Verification items for the finished model (mm, model axes). Face numbers are marked on the shaded views. A direction names the side the tool comes from. Round coordinates to 2 decimals unless told otherwise and drop trailing zeros. Write each loop counter-clockwise with the first axis right and the second up, starting at its lowest first coordinate (ties: lowest second). Pieces come first, ordered by that corner, then holes. Notation, with made-up numbers: (-5.75, 23) - (48.25, 23) arc R17 cw to (48.25, 39) - close; hole circle Ø7 at (83, -23). An arc over 180 degrees is marked (long way). Answer as a JSON object with one key per item and string values.
```python
from build123d import *

# Parameters (mm, degrees)
BOSS_EXTRUDE1_START = 7.7
SKETCH2_R           = 1.295
BOSS_EXTRUDE1_DEPTH = 7.7


with BuildPart() as part:
    # Sketch1 → Revolve1 (revolve)
    with BuildSketch(Plane.XY, mode=Mode.PRIVATE) as revolve1_sk:
        Polygon((-2.7, 0), (-2.7, 5.54), (-1.295, 5.54), (-1.295, 8.3), (-3.32, 8.3), (-3.97, 7.184383121), (-3.97, 3.67), (-4.785, 3.67), (-4.785, 2.47), (-4.28, 2.47), (-4.325, 0), align=None)
    revolve(revolve1_sk.sketch.rotate(Axis((0, 0, 0), (0, 1, 0)), 270), axis=Axis((0, 0, 0), (0, 1, 0)))

    # Sketch2 → Boss-Extrude1 (add)
    with BuildSketch(Plane(origin=(0, 8.3, 0), x_dir=(1, 0, 0), z_dir=(0, 1, 0)).offset(BOSS_EXTRUDE1_START)):
        Polygon((1.799527716, 2.79), (-1.799527716, 2.79), (-2.79, 1.799527716), (-2.79, -1.799527716), (-1.799527716, -2.79), (1.799527716, -2.79), (2.79, -1.799527716), (2.79, 1.799527716), align=None)
        with Locations(Location((0, 0, 0), (0, 0, 90))):
            Circle(SKETCH2_R, mode=Mode.SUBTRACT)
    extrude(amount=-BOSS_EXTRUDE1_DEPTH)


solid = part.part
```
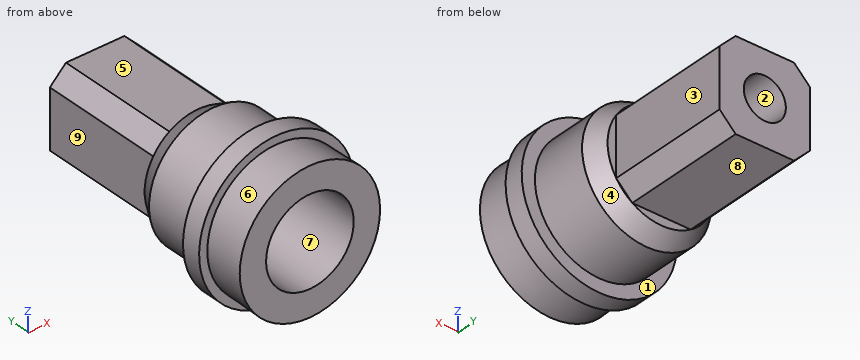
Q1. Section check A-A, the plane y = 8.5. Record the cut outline in (x, z) (3 decimals), then the cut area to 3 significant figures.
Geometry check:
{"outline": "(-2.79, -1.8) - (-1.8, -2.79) - (1.8, -2.79) - (2.79, -1.8) - (2.79, 1.8) - (1.8, 2.79) - (-1.8, 2.79) - (-2.79, 1.8) - close; hole circle Ø2.59 at (0, 0)", "area": "23.9 mm2"}
Q2. Gauge pin test, flat ends, axial feed: P1, Ø1.6, axis at x = 0.5, z = 1, coming from the -Y side; P2, Ø2, axis at x = -1.5, z = -4, coming from the +Y side; P3, Ø2, axis at x = 0.5, y = 9.5, coming from the -Z side. Record the tip position at first contact, or that the pin passes through.
Geometry check:
{"P1": "stops at y = 5.54", "P2": "stops at y = 8.3", "P3": "stops at z = -2.79"}
Q3. Material ranges on line 1 along X through (y, z) = (9.75, 0) (3 decimals); line 2 along X through (y, z) = (3.35, 0) (3 decimals); line 3 along Z through (x, y) = (0.5, 3), recorded low to high. Write a range as [from, to].
Geometry check:
{"line 1": "x = [-2.79, -1.295], [1.295, 2.79]", "line 2": "x = [-4.785, -2.7], [2.7, 4.785]", "line 3": "z = [-4.76, -2.65], [2.65, 4.76]"}
Q4. Set-up check for the marked faces 5, 6, 7, 8 and 9: record each of +Z, -Z, +X, -X, +Y, -Y from which the full face is reachable in a straight line by a thin tool's end or side.
Geometry check:
{"face 5": "+Z, +X, -X, +Y", "face 6": "none", "face 7": "-Y", "face 8": "-Z, +X, -X, +Y", "face 9": "+Z, -Z, -X, +Y"}
Q5. Release check for a two-part mould opening along X. For the marked faces 1, 2, 3 and 4 record: released by +X, released by -X, zero draft, split by the parting line, or undercut.
Geometry check:
{"face 1": "zero draft", "face 2": "undercut", "face 3": "released by +X", "face 4": "split by the parting line"}
